```python
from build123d import *

# Parameters (mm, degrees)
SKETCH_2_W             = 28
SKETCH_2_H             = 4.5
CUT_EXTRUDE_1_DEPTH    = 10
EXTRUDE_1_DEPTH        = 15
HOLE_WIZARD_M3_1_D     = 2.5
HOLE_WIZARD_M3_1_DEPTH = 4
HOLE_WIZARD_M3_1_TIP   = 0.751075774
CUT_EXTRUDE_2_DEPTH    = 20
HOLE_WIZARD_M4_1_D     = 3.3
HOLE_WIZARD_M4_1_DEPTH = 10.1
HOLE_WIZARD_M4_1_TIP   = 0.991420021


with BuildPart() as part:
    # 草图1 → 旋转1 (revolve)
    with BuildSketch(Plane.XY):
        Polygon((0, 0), (4.1, 0), (4.1, 6.7), (13.4, 6.7), (13.4, 8.7), (21, 8.7), (21, 10.2), (20, 10.2), (20, 11.2), (21, 11.2), (21, 12.2), (10, 12.2), (10, 13.2), (21, 13.2), (21, 20.4), (5, 20.4), (5, 21), (21, 21), (21, 34.7), (18.3, 38.7), (3.5, 38.7), (3.5, 43.7), (0, 43.7), align=None)
    revolve(axis=Axis((0, 43.7, 0), (0, -1, 0)))

    # 草图2 → 切除-拉伸1 (cut)
    with BuildSketch(Plane.XY.offset(21)):
        with Locations((0, 16.05)):
            Rectangle(SKETCH_2_W, SKETCH_2_H)
    extrude(amount=-CUT_EXTRUDE_1_DEPTH, mode=Mode.SUBTRACT)

    # 草图3 → 凸台-拉伸1 (add)
    with BuildSketch(Plane.XY.offset(11)):
        with BuildLine():
            Line((9.185056323, 18.053194417), (9.385056323, 18.053194417))
            ThreePointArc((9.385056323, 18.053194417), (11.385056323, 16.053194417), (9.385056323, 14.053194417))
            Line((9.385056323, 14.053194417), (9.185056323, 14.053194417))
            ThreePointArc((9.185056323, 14.053194417), (7.185056323, 16.053194417), (9.185056323, 18.053194417))
        make_face()
    extrude(amount=EXTRUDE_1_DEPTH)

    # M3 螺纹孔1
    with Locations(Plane(origin=(0, 38.7, 0), x_dir=(1, 0, 0), z_dir=(0, 1, 0))):
        with Locations((-6.5, 0), (6.5, 0)):
            Hole(HOLE_WIZARD_M3_1_D / 2, depth=HOLE_WIZARD_M3_1_DEPTH)
            with Locations((0, 0, -(HOLE_WIZARD_M3_1_DEPTH + HOLE_WIZARD_M3_1_TIP / 2))):  # 118° drill point
                Cone(0, HOLE_WIZARD_M3_1_D / 2, HOLE_WIZARD_M3_1_TIP, mode=Mode.SUBTRACT)

    # 草图7 → 旋转2 (revolve)
    with BuildSketch(Plane.XY):
        Polygon((0, -54.6), (5, -54.6), (5, -30.5), (8.275, -30.5), (8.275, -29.6), (13, -29.6), (13, -27.6), (21, -27.6), (21, 8.7), (0, 8.7), align=None)
    revolve(axis=Axis((0, 8.7, 0), (0, -1, 0)))

    # 草图8 → 切除-拉伸2 (cut)
    with BuildSketch(Plane.XZ.offset(54.6)):
        with BuildLine():
            Line((-3, 4), (3, 4))
            ThreePointArc((3, 4), (0, 5), (-3, 4))
        make_face()
    extrude(amount=-CUT_EXTRUDE_2_DEPTH, mode=Mode.SUBTRACT)

    # M4 螺纹孔1
    with Locations(Plane(origin=(0, -27.6, 0), x_dir=(-1, 0, 0), z_dir=(0, -1, 0))):
        with Locations((0, -17.5), (-17.5, 0), (0, 17.5), (17.5, 0)):
            Hole(HOLE_WIZARD_M4_1_D / 2, depth=HOLE_WIZARD_M4_1_DEPTH)
            with Locations((0, 0, -(HOLE_WIZARD_M4_1_DEPTH + HOLE_WIZARD_M4_1_TIP / 2))):  # 118° drill point
                Cone(0, HOLE_WIZARD_M4_1_D / 2, HOLE_WIZARD_M4_1_TIP, mode=Mode.SUBTRACT)


solid = part.part
```
Here's how the part is built. I have some questions about the finished solid (model axes, mm). A direction names the side the tool comes from. Give positions to 0.01 mm unless a question says otherwise; leave off trailing zeros. Write each loop counter-clockwise with the first axis right and the second up, starting at its lowest first coordinate (ties: lowest second). Pieces come first, ordered by that corner, then holes. Notation, with made-up numbers: M -31,87.5 L -26,87.5 A22 cw -26,108.5 Z; hole C 76.5,79.25 d4. An arc over 180 degrees is marked long. Put each result on its own line as item: value. Start each with the question number.
Item 1: On a 3-axis mill with a long thin cutter (end or side, diameter ignored), from which of +Z, -Z, +X, -X, +Y, -Y can I reach the whole of each face in a straight line? I mean faces 1 (the flat face through (9, 16, 26)), 2 (the cylindrical face through (-1.79, -30.04, -8.08)), 3 (the cylindrical face through (11.385, 16.097, 18.395)), 4 (the cylindrical face through (3.233, 41.235, -1.341)), 5 (the flat face through (9, 12.2, 5)). Say none if no direction works.
Item 2: Thinking about a two-plate mould opening in Z: for faces 6 (the flat face through (0, 16, 11)), 7 (the conical face through (-6.72, 34.08, -0.01)), 8 (the flat face through (14, 16, 13)), 9 (the conical face through (0.04, -16.68, 17.22)), which applies, +Z half, -Z half, draft (parallel to the pull), parting line (faces both ways), or undercut?
Item 3: I need wall thicknesses on L1, parallel to Y at x = -2.5, z = 11.5; L2, parallel to Y at x = 14, z = -11; L3, parallel to Y at x = -9, z = 15. Which ranges of each line are inside material? Lowest first, please. Write a range as from..to.
Item 4: If we section it at A-A, the plane y = 27: Write out the boundary of the cut face in (x, z), then the cut area to 3 significant figures.
Item 5: If we section it at B-B, the plane z = -14.5: Count the separate pieces of the cut face and the enclosed holes in it, then the cut area to 3 significant figures.
Item 6: Will these pins go through, and if not, where does the flat tip stop? pin 1 (6 mm diameter, centred on y = 17, z = -16, fed in from +X); pin 2 (1.5 mm diameter, centred on y = -17, z = -10, fed in from +X); pin 3 (2 mm diameter, centred on x = 1, y = -35, fed in from +Z); pin 4 (8 mm diameter, centred on x = -6, z = -1, fed in from -Y).
Values:
1. face 1: +Z, +X, -X, +Y, -Y
1. face 2: -Y
1. face 3: +Z
1. face 4: +Y
1. face 5: none
2. face 6: +Z half
2. face 7: undercut
2. face 8: draft
2. face 9: undercut
3. L1: -29.6..12.2, 13.2..13.8, 18.3..20.4, 21..38.7
3. L2: -27.6..12.2, 13.2..20.4, 21..38.7
3. L3: -27.6..12.2, 13.2..13.8, 18.3..20.4, 21..38.7
4. outline: C 0,0 d42
4. area: 1,390 mm²
5. separate pieces: 3
5. enclosed holes: 0
5. area: 1,950 mm²
6. pin 1: x = 16.49
6. pin 2: x = 18.85
6. pin 3: z = 5
6. pin 4: y = -54.6
